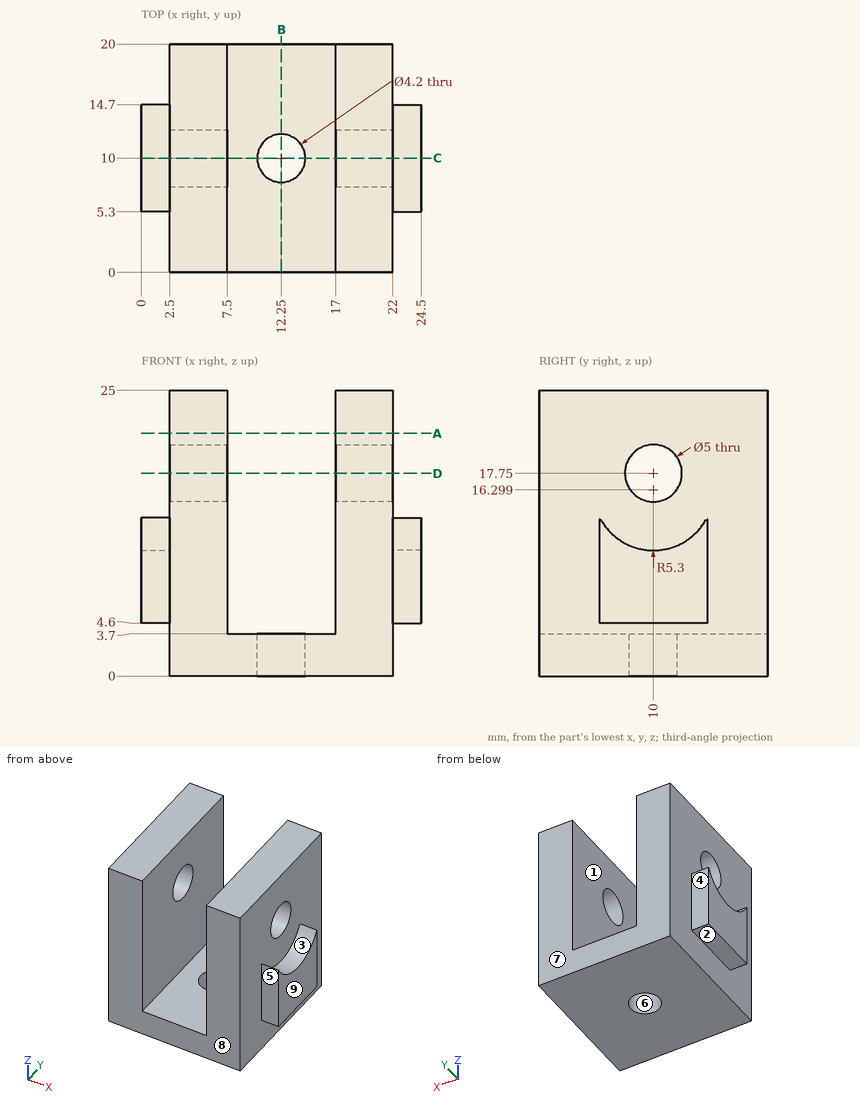
Design review of the part shown in the three views and the two pictorial views. Dimensions are in mm from the part's minimum x, y and z. A direction names the side the tool comes from. Round coordinates to 2 decimals unless told otherwise and drop trailing zeros. Loops run counter-clockwise (first coordinate to the right, second up) from the corner with the lowest first, then second, coordinate; pieces in that order, holes last.
Q1. Add section D-D on z = 17.75. Write out the cut boundary in (x, y), plus the area to 3 significant figures.
Result sheet:
outline: (2.5, 0) - (7.5, 0) - (7.5, 7.5) - (2.5, 7.5) - close; (2.5, 12.5) - (7.5, 12.5) - (7.5, 20) - (2.5, 20) - close; (17, 0) - (22, 0) - (22, 7.5) - (17, 7.5) - close; (17, 12.5) - (22, 12.5) - (22, 20) - (17, 20) - close
area: 150 mm2
Q2. To check wall thickness, follow line 1 along X through (y, z) = (16, 19.75); line 2 along Y through (x, z) = (5.9, 17.75); line 3 along X through (y, z) = (16.5, 1.5). State the ranges of each line that lie inside material, in increasing order.
Result sheet:
line 1: x = 2.5 to 7.5, 17 to 22
line 2: y = 0 to 7.5, 12.5 to 20
line 3: x = 2.5 to 22
Q3. Add section A-A on z = 21.25. Write out the cut boundary in (x, y), plus the area to 3 significant figures.
Result sheet:
outline: (2.5, 0) - (7.5, 0) - (7.5, 20) - (2.5, 20) - close; (17, 0) - (22, 0) - (22, 20) - (17, 20) - close
area: 200 mm2
Q4. Insertion check: pin 1 Ø6.5 at (x, y) = (12.25, 10) entering from +Z; pin 2 Ø2 at (x, z) = (0.5, 7.5) entering from +Y; pin 3 Ø6 at (y, z) = (17, 18) entering from +X. Each pin has a flat end and moves straight along its axis. Give the tip position at first contact, or say it passes through.
Result sheet:
pin 1: stops at z = 3.7
pin 2: stops at y = 14.7
pin 3: stops at x = 22
Q5. Machinability: for the marked faces 1, 2, 3, 4 and 5, which of the approach directions +Z, -Z, +X, -X, +Y, -Y give a long, thin tool a straight path to every point of the face, cutting with its end or side? Answer none if there is none.
Result sheet:
face 1: +Z, +Y, -Y
face 2: -Z, -X, +Y, -Y
face 3: +Z, +X
face 4: +Z, -Z, -X, +Y
face 5: +Z, -Z, +X, -Y
Q6. Add section B-B on x = 12.25. Write out the cut boundary in (y, z).
Result sheet:
outline: (0, 0) - (7.9, 0) - (7.9, 3.7) - (0, 3.7) - close; (12.1, 0) - (20, 0) - (20, 3.7) - (12.1, 3.7) - close
Q7. Mouldability with a two-part tool opening along Y and no side actions: class the marked faces 6, 7, 8 and 9 as +Y half, -Y half, draft (parallel to the pull), parting line (faces both ways), or undercut.
Result sheet:
face 6: undercut
face 7: +Y half
face 8: -Y half
face 9: draft
Q8. Add section C-C on y = 10. Write out the cut boundary in (x, z).
Result sheet:
outline: (0, 4.6) - (2.5, 4.6) - (2.5, 0) - (10.15, 0) - (10.15, 3.7) - (7.5, 3.7) - (7.5, 15.25) - (2.5, 15.25) - (2.5, 11) - (0, 11) - close; (2.5, 20.25) - (7.5, 20.25) - (7.5, 25) - (2.5, 25) - close; (14.35, 0) - (22, 0) - (22, 4.6) - (24.5, 4.6) - (24.5, 11) - (22, 11) - (22, 15.25) - (17, 15.25) - (17, 3.7) - (14.35, 3.7) - close; (17, 20.25) - (22, 20.25) - (22, 25) - (17, 25) - close
